Work out the finished part from the listing and answer in its coordinate system (mm). A direction names the side the tool comes from. Round coordinates to 2 decimals unless told otherwise and drop trailing zeros. Write each loop counter-clockwise with the first axis right and the second up, starting at its lowest first coordinate (ties: lowest second). Pieces come first, ordered by that corner, then holes. Notation, with made-up numbers: M -25,54 L -13,54 A25 ccw -13,69 Z; hole C 21,-3 d10. An arc over 180 degrees is marked long. One line per item, written item: value. Start each with the question number.
Q1. Find section B-B (z = 0). Write down the section's boundary in (x, y).
Q2. Consider probe 1 along X at (y, z) = (10.25, 0); probe 2 along Z at (x, y) = (-2, 8); probe 3 along Z at (x, y) = (-11, 3). Determine where each line is inside the solid, lowest interval first.
Q3. Find section D-D (x = 15). Write down the section's boundary in (y, z).
Q4. The mould has two halves that part along X. Classify faces 1 (the flat face through (0, 4.722, 19)), 2 (the cylindrical face through (-25.861, 6.902, -33.727)), 3 (the flat face through (-9, 0, 9)): released by +X, released by -X, zero draft, split by the parting line, or undercut.
Q5. Find section C-C (y = 11.75). Write down the section's boundary in (x, z), and give its area (3 significant figures).
Q6. A tool of negligible diameter and unlimited length cuts with its end or side. For faces 4 (the cylindrical face through (3.755, 6.902, 11.923)), 5 (the flat face through (19, 4.722, 0)), from which of +Z, -Z, +X, -X, +Y, -Y can it reach the whole face along a straight path? Write none if from no direction.
Q7. Given pin 1 Ø3.5 at (x, z) = (-18.62, 0) entering from +Y; pin 2 Ø5 at (x, y) = (10.5, 12.5) entering from +Z; pin 3 Ø15 at (x, z) = (0, 0) entering from -Y; pin 4 Ø5 at (y, z) = (11.5, 10) entering from -X, each flat-ended and moving along its own axis, determine where each tip first touches the part or whether it passes through.
Q8. Find section A-A (x = 0). Write down the section's boundary in (y, z), and give its area (3 significant figures).
from build123d import *

# Parameters (mm, degrees)
SKETCH1_R             = 42.5
BOSS_EXTRUDE1_DEPTH   = 14
SKETCH2_R             = 12.5
CUT_EXTRUDE1_DEPTH    = 62.713045622
SKETCH3_R             = 2.173069289
CUT_EXTRUDE2_DEPTH    = 9.278215
CIRPATTERN1_START     = 4.721784886
CIRPATTERN1_OUTLINE_R = 2.173069289
CIRPATTERN1_DEPTH     = 9.278215114


# Read off the part's stored shape, not the designer's step: CirPattern1
with BuildPart() as part:
    # Sketch1 → Boss-Extrude1 (new body)
    with BuildSketch(Plane(origin=(0, 0, 0), x_dir=(1, 0, 0), z_dir=(0, 1, 0))):
        with Locations(Location((0, 0, 0), (0, 0, 270))):
            Circle(SKETCH1_R)
    extrude(amount=BOSS_EXTRUDE1_DEPTH)

    # Sketch2 → Cut-Extrude1 (cut, through all)
    with BuildSketch(Plane(origin=(0, 0, 0), x_dir=(1, 0, 0), z_dir=(0, 1, 0))):
        with Locations(Location((0, 0, 0), (0, 0, 270))):
            Circle(SKETCH2_R)
    extrude(amount=CUT_EXTRUDE1_DEPTH, mode=Mode.SUBTRACT)

    # Sketch3 → Cut-Extrude2 (cut)
    with BuildSketch(Plane(origin=(0, 14, 0), x_dir=(1, 0, 0), z_dir=(0, 1, 0))):
        with Locations(Location((-18.619536516, 0, 0), (0, 0, 270))):
            Circle(SKETCH3_R)
    extrude(amount=-CUT_EXTRUDE2_DEPTH, mode=Mode.SUBTRACT)

    # CirPattern1 outline → CirPattern1 (cut)
    with BuildSketch(Plane(origin=(0, 0, 0), x_dir=(1, 0, 0), z_dir=(0, 1, 0)).offset(CIRPATTERN1_START)):
        with Locations((0, 18.619536516)):
            Circle(CIRPATTERN1_OUTLINE_R)
        with Locations((18.619536516, 0)):
            Circle(CIRPATTERN1_OUTLINE_R)
        with Locations((0, -18.619536516)):
            Circle(CIRPATTERN1_OUTLINE_R)
    extrude(amount=CIRPATTERN1_DEPTH, mode=Mode.SUBTRACT)


solid = part.part
The answers:
1. outline: M -42.5,0 L -12.5,0 L -12.5,14 L -16.45,14 L -16.45,4.72 L -20.79,4.72 L -20.79,14 L -42.5,14 Z; M 12.5,0 L 42.5,0 L 42.5,14 L 20.79,14 L 20.79,4.72 L 16.45,4.72 L 16.45,14 L 12.5,14 Z
2. probe 1: -42.5 to -20.79, -16.45 to -12.5, 12.5 to 16.45, 20.79 to 42.5
2. probe 2: -42.45 to -19.47, -17.77 to -12.34, 12.34 to 17.77, 19.47 to 42.45
2. probe 3: -41.05 to -5.94, 5.94 to 41.05
3. outline: M 0,-39.76 L 14,-39.76 L 14,39.76 L 0,39.76 Z
4. face 1: undercut
4. face 2: split by the parting line
4. face 3: zero draft
5. outline: C 0,0 d85; hole C -18.62,0 d4.35; hole C 0,0 d25; hole C 0,-18.62 d4.35; hole C 0,18.62 d4.35; hole C 18.62,0 d4.35
5. area: 5,120 mm2
6. face 4: +Y, -Y
6. face 5: +Y
7. pin 1: y = 4.72
7. pin 2: z = 41.74
7. pin 3: through
7. pin 4: x = -41.83
8. outline: M 0,-42.5 L 14,-42.5 L 14,-20.79 L 4.72,-20.79 L 4.72,-16.45 L 14,-16.45 L 14,-12.5 L 0,-12.5 Z; M 0,12.5 L 14,12.5 L 14,16.45 L 4.72,16.45 L 4.72,20.79 L 14,20.79 L 14,42.5 L 0,42.5 Z
8. area: 759 mm2
